The model under review builds one solid part; all positions refer to its coordinate system, in mm. Face numbers are marked on the shaded views. A direction names the side the tool comes from. Give positions to 0.01 mm unless a question says otherwise; leave off trailing zeros. Loops run counter-clockwise (first coordinate to the right, second up) from the corner with the lowest first, then second, coordinate; pieces in that order, holes last. Notation, with made-up numbers: M 3.5,11 L 23.5,11 A24 cw 23.5,41 Z; hole C 22.5,-30 d11. An arc over 180 degrees is marked long. One line per item, written item: value. Start each with the question number.
Q1. We need section A-A on z = 5. Write out the cut boundary in (x, y), plus the area to 3 significant figures.
Q2. We need section B-B on x = -21. Write out the cut boundary in (y, z), plus the area to 3 significant figures.
Q3. For the marked faces 1 and 2, list the 3-axis set-ups (+Z, -Z, +X, -X, +Y, -Y) from which the entire face can be reached by the end or side of a thin tool; tool diameter is ignored.
Q4. Mouldability with a two-part tool opening along Z and no side actions: class the marked faces 3, 4, 5 and 6 as released by +Z, released by -Z, zero draft, split by the parting line, or undercut.
Q5. We need section C-C on y = -2.6. Write out the cut boundary in (x, z), plus the area to 3 significant figures.
Q6. To check wall thickness, follow line 1 along X through (y, z) = (-1.25, 4.25); line 2 along X through (y, z) = (-3.85, 1.75); line 3 along Z through (x, y) = (-9.5, -2.1). State the ranges of each line that lie inside material, in increasing order. Write a range as from..to.
```python
from build123d import *

# Parameters (mm, degrees)
F0_W     = 49
F0_H     = 17
F0_W_2   = 2.5
F0_H_2   = 11
F1_DEPTH = 5
F3_D     = 3.2
F4_R     = 2


with BuildPart() as f1:
    # F0 (on Front) → F1 (new body)
    with BuildSketch(Plane.XZ):
        Rectangle(F0_W, F0_H)
        with Locations((-9, -1.5)):
            Rectangle(F0_W_2, F0_H_2, mode=Mode.SUBTRACT)
        with Locations((-4.5, -1.5)):
            Rectangle(F0_W_2, F0_H_2, mode=Mode.SUBTRACT)
        with Locations((4.5, 1.5)):
            Rectangle(F0_W_2, F0_H_2, mode=Mode.SUBTRACT)
        with Locations((9, 1.5)):
            Rectangle(F0_W_2, F0_H_2, mode=Mode.SUBTRACT)
    extrude(amount=F1_DEPTH)

    # F3 (through all)
    with Locations(Plane(origin=(0, 0, 0), x_dir=(1, 0, 0), z_dir=(0, 1, 0))):
        with Locations((-21, 0), (21, 0)):
            Hole(F3_D / 2)

    # F4
    f4_edges = [f1.edges().sort_by_distance(p)[0] for p in [
        (-24.5, -2.5, 8.5),
        (-24.5, -2.5, -8.5),
        (24.5, -2.5, 8.5),
        (24.5, -2.5, -8.5),
    ]]
    fillet(f4_edges, radius=F4_R)


solid = f1.part
```
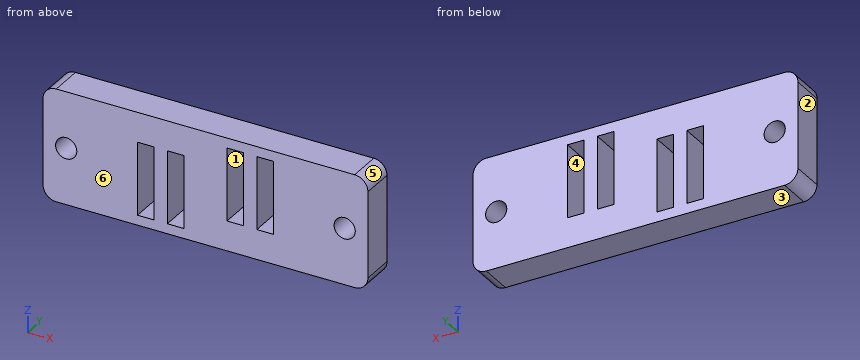
Solved:
1. outline: M -24.5,-5 L 3.25,-5 L 3.25,0 L -24.5,0 Z; M 5.75,-5 L 7.75,-5 L 7.75,0 L 5.75,0 Z; M 10.25,-5 L 24.5,-5 L 24.5,0 L 10.25,0 Z
1. area: 220 mm2
2. outline: M -5,-8.5 L 0,-8.5 L 0,-1.6 L -5,-1.6 Z; M -5,1.6 L 0,1.6 L 0,8.5 L -5,8.5 Z
2. area: 69.0 mm2
3. face 1: +Y, -Y
3. face 2: +Z, -Z, -X, +Y, -Y
4. face 3: released by -Z
4. face 4: undercut
4. face 5: released by +Z
4. face 6: zero draft
5. outline: M -24.5,-6.5 A2 ccw -22.5,-8.5 L 22.5,-8.5 A2 ccw 24.5,-6.5 L 24.5,6.5 A2 ccw 22.5,8.5 L -22.5,8.5 A2 ccw -24.5,6.5 Z; hole C -21,0 d3.2; hole M -10.25,-7 L -7.75,-7 L -7.75,4 L -10.25,4 Z; hole M -5.75,-7 L -3.25,-7 L -3.25,4 L -5.75,4 Z; hole M 3.25,-4 L 5.75,-4 L 5.75,7 L 3.25,7 Z; hole M 7.75,-4 L 10.25,-4 L 10.25,7 L 7.75,7 Z; hole C 21,0 d3.2
5. area: 703 mm2
6. line 1: -24.5..3.25, 5.75..7.75, 10.25..24.5
6. line 2: -24.5..-10.25, -7.75..-5.75, -3.25..3.25, 5.75..7.75, 10.25..24.5
6. line 3: -8.5..-7, 4..8.5
